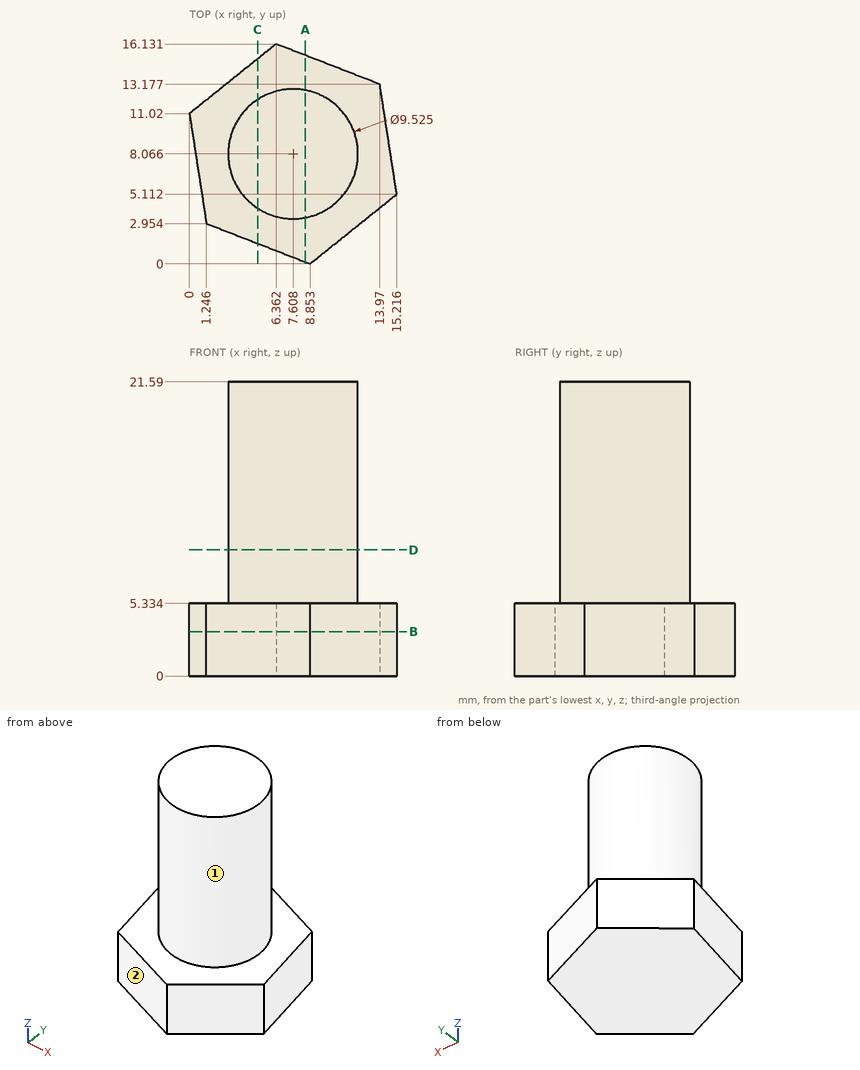
Print and shaded views of the part. All mm, measured from the part's lowest x, y and z. A direction names the side the tool comes from. Round coordinates to 2 decimals unless told otherwise and drop trailing zeros. Order: outer loops, then holes, each group sorted by start corner. A loop starts at its lowest first (then second) coordinate and runs counter-clockwise, first axis right, second up. Notation, with made-up numbers: (33.25, 53.25) - (75.25, 53.25) arc R5 ccw to (75.25, 57.25) - close; hole circle Ø11 at (-25, -7). An arc over 180 degrees is marked (long way). Use a Markdown table: item, result.
1) Wall check: L1, parallel to Z at x = 2.25, y = 3; L2, parallel to X at y = 3.5, z = 2.25; L3, parallel to Y at x = 10, z = 19.75 (1 decimal). Give the ranges that are in metal, low to high.
Recorded:
| item | result |
|---|---|
| L1 | z = 0 to 5.33 |
| L2 | x = 1.16 to 13.21 |
| L3 | y = 3.9 to 12.2 |
2) Saw through at D-D on z = 9.25. Write the cut outline in (x, y) (1 decimal).
Recorded:
| item | result |
|---|---|
| outline | circle Ø9.5 at (7.6, 8.1) |
3) Tool access for the marked faces 1 and 2: list every direction of +Z, -Z, +X, -X, +Y, -Y with a clear straight run to the whole face (end or side of a thin tool).
Recorded:
| item | result |
|---|---|
| face 1 | +Z |
| face 2 | +Z, -Z, -X, -Y |
4) Saw through at A-A on x = 8.5. Write the cut outline in (y, z).
Recorded:
| item | result |
|---|---|
| outline | (0.14, 0) - (15.3, 0) - (15.3, 5.33) - (12.74, 5.33) - (12.74, 21.59) - (3.39, 21.59) - (3.39, 5.33) - (0.14, 5.33) - close |
5) Saw through at B-B on z = 3.25. Write the cut outline in (x, y) (1 decimal).
Recorded:
| item | result |
|---|---|
| outline | (0, 11) - (1.2, 3) - (8.9, 0) - (15.2, 5.1) - (14, 13.2) - (6.4, 16.1) - close |
6) Flat gauge pins, fed straight in: pin 1 Ø4 at (y, z) = (4, 18.5) entering from -X; pin 2 Ø6 at (y, z) = (2.5, 5.5) entering from -X; pin 3 Ø2 at (y, z) = (11.5, 13) entering from +X. Where does each tip first touch, or does it go through?
Recorded:
| item | result |
|---|---|
| pin 1 | stops at x = 3.32 |
| pin 2 | stops at x = 0.85 |
| pin 3 | stops at x = 11.7 |
7) Saw through at C-C on x = 5. Write the cut outline in (y, z), and give its area (3 significant figures).
Recorded:
| item | result |
|---|---|
| outline | (1.5, 0) - (15.04, 0) - (15.04, 5.33) - (12.05, 5.33) - (12.05, 21.59) - (4.08, 21.59) - (4.08, 5.33) - (1.5, 5.33) - close |
| area | 202 mm² |
